Input: part model. Units: mm. Frame: model coordinates. Coordinates: 2 decimals unless noted, no trailing zeros. Order: outer loops, then holes, each group sorted by start corner. A loop starts at its lowest first (then second) coordinate and runs counter-clockwise, first axis right, second up. Notation, with made-up numbers: (68.25, 84) -> (100.25, 84) arc R20 cw to (100.25, 116) -> close; hole circle Ø4 at (39.5, -30). An arc over 180 degrees is marked (long way). Use one line per item in the form item = value. Start each with the question number.
1) Draft query along Z for faces 1 (the flat face through (0, 1, -18.5)), 2 (the flat face through (-28.5, 1, 0)), 3 (the cylindrical face through (-24.92, 0.85, -17.18)), 4 (the flat face through (0, 1, 18.5)). Return one class per face: pulls with the +Z half, pulls with the -Z half, needs draft (parallel to the pull), parting line crosses it, or undercut.
2) Section query A-A on z = -6.04. Output: boundary loops of the cut face in (x, y), then the cut area to 3 significant figures.
3) Ray query, line 1 along X through (y, z) = (0.85, 16); line 2 along X through (y, z) = (0.45, 4.63); line 3 along Z through (x, y) = (-14, 0.7). Return the intervals inside material, ascending.
4) Section query B-B on y = 0.85. Output: boundary loops of the cut face in (x, z).
5) Section query C-C on x = -13.4. Output: boundary loops of the cut face in (y, z).
6) Section query D-D on z = -16. Output: boundary loops of the cut face in (x, y).
from build123d import *

# Parameters (mm, degrees)
SKETCH1_W           = 57
SKETCH1_H           = 37
BOSS_EXTRUDE1_DEPTH = 1.67
SKETCH2_R           = 1.6
CUT_EXTRUDE1_DEPTH  = 1.67


with BuildPart() as part:
    # Sketch1 → Boss-Extrude1 (new body)
    with BuildSketch(Plane(origin=(0, 0, 0), x_dir=(1, 0, 0), z_dir=(0, 1, 0))):
        Rectangle(SKETCH1_W, SKETCH1_H)
    extrude(amount=BOSS_EXTRUDE1_DEPTH)

    # Sketch2 → Cut-Extrude1 (cut)
    with BuildSketch(Plane(origin=(0, 1.67, 0), x_dir=(1, 0, 0), z_dir=(0, 1, 0))):
        with Locations(Location((-26, -16, 0), (0, 0, 270))):
            Circle(SKETCH2_R)
        with Locations(Location((-26, 16, 0), (0, 0, 270))):
            Circle(SKETCH2_R)
        with Locations(Location((26, -16, 0), (0, 0, 270))):
            Circle(SKETCH2_R)
        with Locations(Location((26, 16, 0), (0, 0, 270))):
            Circle(SKETCH2_R)
        with Locations(Location((-13.4, 6.04, 0), (0, 0, 270))):
            Circle(SKETCH2_R)
        with Locations(Location((-21.81, -4.63, 0), (0, 0, 270))):
            Circle(SKETCH2_R)
    extrude(amount=-CUT_EXTRUDE1_DEPTH, mode=Mode.SUBTRACT)


solid = part.part
Answers below:
q1.face_1 = pulls with the -Z half
q1.face_2 = needs draft
q1.face_3 = undercut
q1.face_4 = pulls with the +Z half
q2.outline = (-28.5, 0) -> (-15, 0) -> (-15, 1.67) -> (-28.5, 1.67) -> close; (-11.8, 0) -> (28.5, 0) -> (28.5, 1.67) -> (-11.8, 1.67) -> close
q2.area = 89.8 mm^2
q3.line_1 = -28.5 to -27.6, -24.4 to 24.4, 27.6 to 28.5
q3.line_2 = -28.5 to -23.41, -20.21 to 28.5
q3.line_3 = -18.5 to -7.52, -4.56 to 18.5
q4.outline = (-28.5, -18.5) -> (28.5, -18.5) -> (28.5, 18.5) -> (-28.5, 18.5) -> close; hole circle Ø3.2 at (-26, -16); hole circle Ø3.2 at (-26, 16); hole circle Ø3.2 at (-21.81, 4.63); hole circle Ø3.2 at (-13.4, -6.04); hole circle Ø3.2 at (26, -16); hole circle Ø3.2 at (26, 16)
q5.outline = (0, -18.5) -> (1.67, -18.5) -> (1.67, -7.64) -> (0, -7.64) -> close; (0, -4.44) -> (1.67, -4.44) -> (1.67, 18.5) -> (0, 18.5) -> close
q6.outline = (-28.5, 0) -> (-27.6, 0) -> (-27.6, 1.67) -> (-28.5, 1.67) -> close; (-24.4, 0) -> (24.4, 0) -> (24.4, 1.67) -> (-24.4, 1.67) -> close; (27.6, 0) -> (28.5, 0) -> (28.5, 1.67) -> (27.6, 1.67) -> close
